```python
from build123d import *

# Parameters (mm, degrees)
SKETCH_R      = 22.5
SKETCH_R_2    = 8
PAD_DEPTH     = 15
SKETCH002_R   = 35
SKETCH002_R_2 = 22.5
PAD001_DEPTH  = 20


with BuildPart() as part:
    # Sketch → Pad (new body)
    with BuildSketch(Plane.XY):
        with BuildLine():
            ThreePointArc((9.5455310911, 33.6731768057), (3.97682e-05, 35), (-9.5454545699, 33.6731984975))
            Line((-60.4545457907, 19.2418276215), (-9.5454545698, 33.6731984975))
            ThreePointArc((-60.4545457907, 19.2418276215), (-75, -1.844e-07), (-60.4545454359, -19.2418277221))
            Line((-60.4545454359, -19.2418277221), (-9.5454544023, -33.673198545))
            ThreePointArc((-9.5454544023, -33.673198545), (3.842e-07, -35), (9.5454551416, -33.6731983355))
            Line((9.5454551416, -33.6731983355), (60.4545455403, -19.2418276925))
            ThreePointArc((60.4545455403, -19.2418276925), (75, 6.189e-07), (60.4545443494, 19.2418280301))
            Line((9.5455310911, 33.6731768057), (60.4545443495, 19.2418280301))
        make_face()
        Circle(SKETCH_R, mode=Mode.SUBTRACT)
        with Locations((-55, 0)):
            Circle(SKETCH_R_2, mode=Mode.SUBTRACT)
        with Locations((55, 0)):
            Circle(SKETCH_R_2, mode=Mode.SUBTRACT)
    extrude(amount=PAD_DEPTH)

    # Sketch002 → Pad001 (new body)
    with BuildSketch(Plane.XY.offset(15)):
        Circle(SKETCH002_R)
        Circle(SKETCH002_R_2, mode=Mode.SUBTRACT)
    extrude(amount=PAD001_DEPTH)


solid = part.part
```
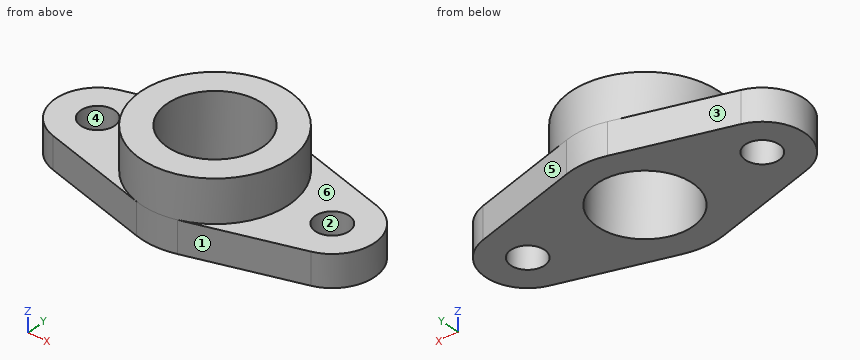
The listing builds one solid part. Answer for the finished solid, in the listing's coordinates (mm). Face numbers are marked on the shaded views. A direction names the side the tool comes from. Coordinates: 2 decimals unless noted, no trailing zeros. Loops run counter-clockwise (first coordinate to the right, second up) from the corner with the lowest first, then second, coordinate; pieces in that order, holes last. Notation, with made-up numbers: (15, -36) -> (39, -36) arc R21 ccw to (39, -22) -> close; hole circle Ø10 at (81.5, 17). An arc over 180 degrees is marked (long way). Use one line per item in the form item = value. Start each with the question number.
Item 1: The mould has two halves that part along Y. Classify the marked faces 1, 2, 3 and 4: released by +Y, released by -Y, zero draft, split by the parting line, or undercut.
Item 2: Flat-ended cylindrical pins translate along their axes: pin 1 Ø10 at (x, z) = (21, 7) entering from -Y; pin 2 Ø21 at (x, y) = (-55, 0) entering from +Z; pin 3 Ø2 at (x, z) = (-25, 9) entering from +Y. Find the tip coordinate at first contact, or state that the pin passes through.
Item 3: Consider L1, parallel to Y at x = 0, z = 24; L2, parallel to X at y = -7, z = 20; L3, parallel to X at y = -16.5, z = 12. Determine where each line is inside the solid, lowest interval first. Write a range as [from, to].
Item 4: The part is cut by section D-D on y = 15. Determine the outline of the cut face in (x, z), then the cut area to 3 significant figures.
Item 5: The part is cut by section C-C on z = 3.5. Determine the outline of the cut face in (x, y), then the cut area to 3 significant figures.
Item 6: A tool of negligible diameter and unlimited length cuts with its end or side. For the marked faces 5 and 6, from which of +Z, -Z, +X, -X, +Y, -Y can it reach the whole face along a straight path? Write none if from no direction.
Item 7: The part is cut by section B-B on y = 0. Determine the outline of the cut face in (x, z), then the cut area to 4 significant figures.
Item 8: The part is cut by section A-A on x = 0. Determine the outline of the cut face in (y, z).
Answer key:
q1.face_1 = released by -Y
q1.face_2 = undercut
q1.face_3 = released by +Y
q1.face_4 = undercut
q2.pin_1 = -31.84
q2.pin_2 = 15
q2.pin_3 = 29.58
q3.L1 = [-35, -22.5], [22.5, 35]
q3.L2 = [-34.29, -21.38], [21.38, 34.29]
q3.L3 = [-66.3, -15.3], [15.3, 66.3]
q4.outline = (-68.23, 0) -> (-16.77, 0) -> (-16.77, 35) -> (-31.62, 35) -> (-31.62, 15) -> (-68.23, 15) -> close; (16.77, 0) -> (68.23, 0) -> (68.23, 15) -> (31.62, 15) -> (31.62, 35) -> (16.77, 35) -> close
q4.area = 2,140 mm2
q5.outline = (-60.45, -19.24) -> (-9.55, -33.67) arc R35 ccw to (9.55, -33.67) -> (60.45, -19.24) arc R20 ccw to (60.45, 19.24) -> (9.55, 33.67) arc R35 ccw to (-9.55, 33.67) -> (-60.45, 19.24) arc R20 ccw to start; hole circle Ø16 at (-55, 0); hole circle Ø45 at (0, 0); hole circle Ø16 at (55, 0)
q5.area = 5,540 mm2
q6.face_5 = +Z, -Z, +X, +Y
q6.face_6 = +Z, +X
q7.outline = (-75, 0) -> (-63, 0) -> (-63, 15) -> (-75, 15) -> close; (-47, 0) -> (-22.5, 0) -> (-22.5, 35) -> (-35, 35) -> (-35, 15) -> (-47, 15) -> close; (22.5, 0) -> (47, 0) -> (47, 15) -> (35, 15) -> (35, 35) -> (22.5, 35) -> close; (63, 0) -> (75, 0) -> (75, 15) -> (63, 15) -> close
q7.area = 1,595 mm2
q8.outline = (-35, 0) -> (-22.5, 0) -> (-22.5, 35) -> (-35, 35) -> close; (22.5, 0) -> (35, 0) -> (35, 35) -> (22.5, 35) -> close
